from build123d import *

# Parameters (mm, degrees)
SKETCH1_R           = 3.7084
SKETCH1_W           = 1.778
SKETCH1_H           = 1.5875
SKETCH1_W_2         = 1.5875
SKETCH1_H_2         = 1.3208
BOSS_EXTRUDE1_DEPTH = 1.5875


with BuildPart() as part:
    # Sketch1 → Boss-Extrude1 (new body)
    # profile 1 of 4: a face of its own
    with BuildSketch(Plane.XY):
        with BuildLine():
            Line((-10.431265191, -4.028360607), (-2.823309713, -4.028360607))
            Line((-2.823309713, -4.028360607), (12.7, -2.670246987))
            Line((12.7, -2.670246987), (12.7, 16.51))
            Line((12.7, 16.51), (10.10362126, 16.51))
            Line((10.10362126, 16.51), (8.32562126, 16.51))
            Line((8.32562126, 16.51), (-4.89637874, 16.51))
            Line((-4.89637874, 16.51), (-6.67437874, 16.51))
            Line((-6.67437874, 16.51), (-7.62, 16.51))
            ThreePointArc((-7.62, 16.51), (-10.314076836, 15.394076836), (-11.43, 12.7))
            Line((-11.43, 12.7), (-11.43, 1.3208))
            Line((-11.43, 1.3208), (-11.43, 0))
            Line((-11.43, 0), (-11.43, -2.009424845))
            ThreePointArc((-11.43, -2.009424845), (-11.166665718, -3.135654487), (-10.431265191, -4.028360607))
        make_face()
        Circle(SKETCH1_R, mode=Mode.SUBTRACT)
        with BuildLine():
            ThreePointArc((-3.82905, 11.642311449), (4.572, 9.144), (-3.82905, 6.645688551))
            ThreePointArc((-3.82905, 6.645688551), (-7.874, 9.144), (-3.82905, 11.642311449))
        make_face(mode=Mode.SUBTRACT)
    # profile 2 of 4: a face of its own
    with BuildSketch(Plane.XY):
        with Locations((-5.78537874, 17.30375)):
            Rectangle(SKETCH1_W, SKETCH1_H)
    # profile 3 of 4: a face of its own
    with BuildSketch(Plane.XY):
        with Locations((9.21462126, 17.30375)):
            Rectangle(SKETCH1_W, SKETCH1_H)
    # profile 4 of 4: a face of its own
    with BuildSketch(Plane.XY):
        with Locations((-12.22375, 0.6604)):
            Rectangle(SKETCH1_W_2, SKETCH1_H_2)
    extrude(amount=BOSS_EXTRUDE1_DEPTH)


solid = part.part
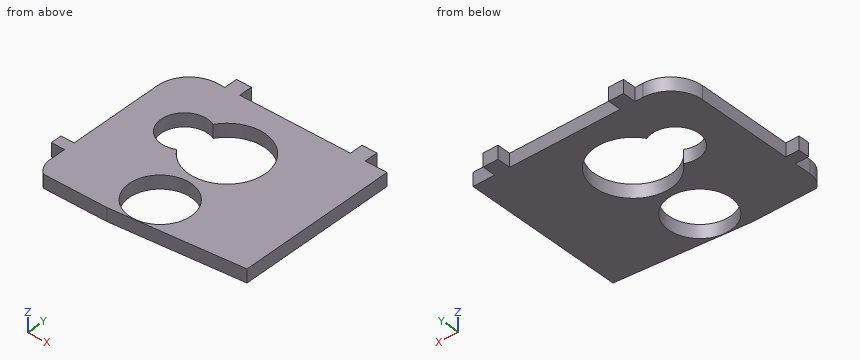
Model file for the job. Use its own axes, mm. Give positions to 0.01 mm unless a question says otherwise; leave off trailing zeros. Write each loop counter-clockwise with the first axis right and the second up, starting at its lowest first coordinate (ties: lowest second). Pieces come first, ordered by that corner, then holes. Notation, with made-up numbers: M 3,-23 L 12,-23 A29 ccw 12,15 Z; hole C 12,-21 d8. An arc over 180 degrees is marked long. One line per item, written item: value. Start each with the question number.
Q1. Saw through at C-C, the plane z = 0.95. Write the cut outline in (x, y), plus the area to 3 significant figures.
Q2. Probe probe 1 along Y at (x, z) = (-5.08, 1.15); probe 2 along X at (y, z) = (9, 0.3); probe 3 along Y at (x, z) = (-2, 1.45). List the from-to ranges inside material, lowest first. Write a range as [from, to].
Q3. Saw through at D-D, the plane x = 3.25. Write the cut outline in (y, z), plus the area to 3 significant figures.
Q4. Drop flat-ended pins along their axis: pin 1 Ø0.8 at (x, z) = (-12.5, 1) entering from +Y; pin 2 Ø0.8 at (y, z) = (17, 1) entering from +X; pin 3 Ø0.5 at (y, z) = (8, 1) entering from -X. Give the stop position or say it passes through.
Q5. Saw through at B-B, the plane x = 0. Write the cut outline in (y, z), plus the area to 3 significant figures.
Q6. Saw through at A-A, the plane y = 9.25. Write the cut outline in (x, z).
Output values:
1. outline: M -13.02,0 L -11.43,0 L -11.43,-2.01 A2.54 ccw -10.43,-4.03 L -2.82,-4.03 L 12.7,-2.67 L 12.7,16.51 L 10.1,16.51 L 10.1,18.1 L 8.33,18.1 L 8.33,16.51 L -4.9,16.51 L -4.9,18.1 L -6.67,18.1 L -6.67,16.51 L -7.62,16.51 A3.81 ccw -11.43,12.7 L -11.43,1.32 L -13.02,1.32 Z; hole M -3.83,6.65 A4.57 ccw long -3.83,11.64 A2.79 ccw long Z; hole C 0,0 d7.42
1. area: 364 mm²
2. probe 1: y = [-4.03, 6.35], [11.94, 18.1]
2. probe 2: x = [-11.43, -7.87], [4.57, 12.7]
2. probe 3: y = [-3.96, -3.12], [3.12, 5.03], [13.26, 16.51]
3. outline: M -3.5,0 L -1.79,0 L -1.79,1.59 L -3.5,1.59 Z; M 1.79,0 L 5.93,0 L 5.93,1.59 L 1.79,1.59 Z; M 12.36,0 L 16.51,0 L 16.51,1.59 L 12.36,1.59 Z
3. area: 15.9 mm²
4. pin 1: stops at y = 1.32
4. pin 2: stops at x = 10.1
4. pin 3: stops at x = -11.43
5. outline: M -3.78,0 L -3.71,0 L -3.71,1.59 L -3.78,1.59 Z; M 3.71,0 L 4.57,0 L 4.57,1.59 L 3.71,1.59 Z; M 13.72,0 L 16.51,0 L 16.51,1.59 L 13.72,1.59 Z
5. area: 5.92 mm²
6. outline: M -11.43,0 L -7.87,0 L -7.87,1.59 L -11.43,1.59 Z; M 4.57,0 L 12.7,0 L 12.7,1.59 L 4.57,1.59 Z
